Verification items for the finished model (mm, model axes). Face numbers are marked on the shaded views. A direction names the side the tool comes from. Give positions to 0.01 mm unless a question says otherwise; leave off trailing zeros. Write each loop counter-clockwise with the first axis right and the second up, starting at its lowest first coordinate (ties: lowest second). Pieces come first, ordered by that corner, then holes. Notation, with made-up numbers: (56, 60.25) - (74, 60.25) arc R14 ccw to (74, 69.25) - close; hole circle Ø7 at (-38, 61). An arc over 180 degrees is marked (long way). Answer as a JSON object with one key per item and string values. Group by question number.
Item 1: Sectioned sample at B-B, the plane x = 0. Record the boundary of the cut face in (y, z), and give its area (3 significant figures).
Item 2: Sectioned sample at C-C, the plane y = 0. Record the boundary of the cut face in (x, z), and give its area (3 significant figures).
Item 3: Draft check along Z on the marked faces 4 and 5. Enter one of: +Z half, -Z half, draft (parallel to the pull), parting line (faces both ways), or undercut.
Item 4: Tool access check on the marked faces 1, 2 and 3. Record the directions out of +Z, -Z, +X, -X, +Y, -Y that give a thin tool (end or side, any length) a straight path to the whole face; none if there is none.
Item 5: Scan lines: line 1 along Y through (x, z) = (-19.5, 11.5); line 2 along Y through (x, z) = (-3, -15); line 3 along Y through (x, z) = (19, 4). Record each from-to range of solid material in increasing order. Write a range as [from, to].
Item 6: Go/stop test with flat-tipped pins: pin 1 (17 mm diameter, centred on x = 0, z = 0, fed in from -Y); pin 2 (3 mm diameter, centred on x = -17, y = 3.5, fed in from +Z); pin 3 (3 mm diameter, centred on y = -0.5, z = 12, fed in from +X); pin 4 (15 mm diameter, centred on x = -4.5, z = 10.5, fed in from +Y). Record where each tip stops, or that it passes through.
Item 7: Sectioned sample at A-A, the plane z = 0. Record the boundary of the cut face in (x, y), and give its area (3 significant figures).
```python
from build123d import *


with BuildPart() as part:
    # Эскиз1 → Повернуть1 (revolve)
    with BuildSketch(Plane.XY):
        with BuildLine():
            Line((7.5, 4), (7.5, -4))
            Line((7.5, -4), (15.93289357, -4))
            Line((15.93289357, -4), (17.26104157, -6.459147259))
            Line((17.26104157, -6.459147259), (25, -6.459147259))
            Line((25, -6.459147259), (25, -4))
            Line((25, -4), (22, -4))
            ThreePointArc((22, -4), (18, 0), (22, 4))
            Line((22, 4), (25, 4))
            Line((25, 4), (25, 6.459147259))
            Line((25, 6.459147259), (17.26104157, 6.459147259))
            Line((17.26104157, 6.459147259), (15.93289357, 4))
            Line((15.93289357, 4), (7.5, 4))
        make_face()
    revolve(axis=Axis((0, 40.932480583, 0), (0, -1, 0)))


solid = part.part
```
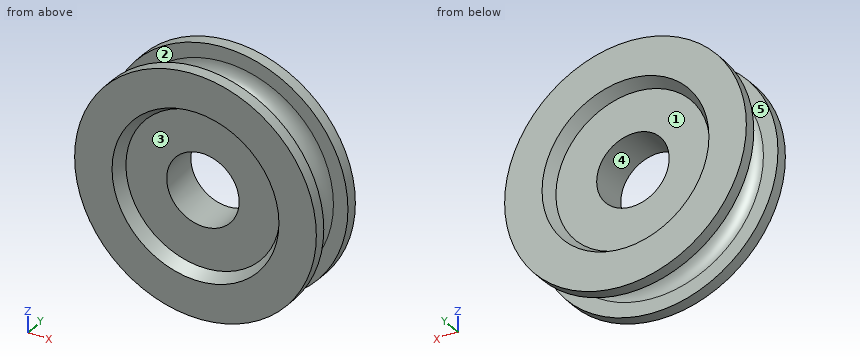
Geometry check:
{
 "1": {"outline": "(-6.46, -25) - (-4, -25) - (-4, -22) arc R4 cw to (4, -22) - (4, -25) - (6.46, -25) - (6.46, -17.26) - (4, -15.93) - (4, -7.5) - (-4, -7.5) - (-4, -15.93) - (-6.46, -17.26) - close; (-6.46, 17.26) - (-4, 15.93) - (-4, 7.5) - (4, 7.5) - (4, 15.93) - (6.46, 17.26) - (6.46, 25) - (4, 25) - (4, 22) arc R4 cw to (-4, 22) - (-4, 25) - (-6.46, 25) - close", "area": "264 mm^2"},
 "2": {"outline": "circle Ø36 at (0, 0); hole circle Ø15 at (0, 0)", "area": "841 mm^2"},
 "3": {"face 4": "undercut", "face 5": "draft"},
 "4": {"face 1": "+Y", "face 2": "none", "face 3": "-Y"},
 "5": {"line 1": "[-6.46, -4], [4, 6.46]", "line 2": "[-4, 4]", "line 3": "[-6.46, -3.05], [3.05, 6.46]"},
 "6": {"pin 1": "y = -4", "pin 2": "z = 19.55", "pin 3": "x = 14.72", "pin 4": "y = 6.46"},
 "7": {"outline": "(-25, -6.46) - (-17.26, -6.46) - (-15.93, -4) - (-7.5, -4) - (-7.5, 4) - (-15.93, 4) - (-17.26, 6.46) - (-25, 6.46) - (-25, 4) - (-22, 4) arc R4 cw to (-22, -4) - (-25, -4) - close; (7.5, -4) - (15.93, -4) - (17.26, -6.46) - (25, -6.46) - (25, -4) - (22, -4) arc R4 cw to (22, 4) - (25, 4) - (25, 6.46) - (17.26, 6.46) - (15.93, 4) - (7.5, 4) - close", "area": "264 mm^2"}
}
